Design review of the part built by this model. Coordinates are the model's own, in mm. A direction names the side the tool comes from. Round coordinates to 2 decimals unless told otherwise and drop trailing zeros. Order: outer loops, then holes, each group sorted by start corner. A loop starts at its lowest first (then second) coordinate and runs counter-clockwise, first axis right, second up. Notation, with made-up numbers: (66.25, 34.25) - (110.25, 34.25) arc R27 ccw to (110.25, 55.25) - close; hole circle Ø10 at (28, -9). An arc over 180 degrees is marked (long way). Write item = value, one per line.
from build123d import *

# Parameters (mm, degrees)
F0_W     = 152.4
F0_H     = 152.4
F1_DEPTH = 152.4
F2_R     = 12.7
F4_D     = 38.1
F5_W     = 57.1246
F5_H     = 22.6568
F6_DEPTH = 152.401


with BuildPart() as f1:
    # F0 (on Front) → F1 (new body)
    with BuildSketch(Plane.XZ):
        with Locations((76.2, 76.2)):
            Rectangle(F0_W, F0_H)
    extrude(amount=F1_DEPTH)

    # F2
    f2_edges = [f1.edges().sort_by_distance(p)[0] for p in [
        (76.2, -152.4, 152.4),
        (0, -76.2, 152.4),
        (76.2, 0, 152.4),
        (152.4, -76.2, 152.4),
    ]]
    fillet(f2_edges, radius=F2_R)

    # F4 (through all)
    with Locations(Plane.YZ.offset(152.4)):
        with Locations((-73.099315, 71.219265)):
            Hole(F4_D / 2)

    # F5 (on face) → F6 (cut, through all)
    with BuildSketch(Plane.XZ.offset(152.4)):
        with Locations((66.187836, 65.461391)):
            Rectangle(F5_W, F5_H)
    extrude(amount=-F6_DEPTH, mode=Mode.SUBTRACT)


solid = f1.part
1) We need section A-A on y = -35. Write out the cut boundary in (x, z), and give its area (3 significant figures).
Findings:
outline = (0, 0) - (152.4, 0) - (152.4, 139.7) arc R12.7 ccw to (139.7, 152.4) - (12.7, 152.4) arc R12.7 ccw to (0, 139.7) - close; hole (37.63, 54.13) - (94.75, 54.13) - (94.75, 76.79) - (37.63, 76.79) - close
area = 21,900 mm^2
2) We need section B-B on x = 59. Write out the cut boundary in (y, z), and give its area (3 significant figures).
Findings:
outline = (-152.4, 0) - (0, 0) - (0, 54.13) - (-64.68, 54.13) arc R19.05 cw to (-81.52, 54.13) - (-152.4, 54.13) - close; (-152.4, 76.79) - (-91.32, 76.79) arc R19.05 cw to (-54.88, 76.79) - (0, 76.79) - (0, 139.7) arc R12.7 ccw to (-12.7, 152.4) - (-139.7, 152.4) arc R12.7 ccw to (-152.4, 139.7) - close
area = 19,300 mm^2
3) We need section D-D on y = -74.5. Write out the cut boundary in (x, z), and give its area (3 significant figures).
Findings:
outline = (0, 0) - (152.4, 0) - (152.4, 52.22) - (0, 52.22) - close; (0, 90.22) - (152.4, 90.22) - (152.4, 139.7) arc R12.7 ccw to (139.7, 152.4) - (12.7, 152.4) arc R12.7 ccw to (0, 139.7) - close
area = 17,400 mm^2
4) To check wall thickness, follow L1, parallel to Z at x = 39, y = -123; L2, parallel to Z at x = 37, y = -82; L3, parallel to Y at x = 16, z = 78.5. State the ranges of each line that lie inside material, in increasing order. Write a range as from..to.
Findings:
L1 = 0..54.13, 76.79..152.4
L2 = 0..54.38, 88.06..152.4
L3 = -152.4..-90.7, -55.5..0
5) The part is to be moulded in two halves that separate along Z. For faces 3 (the flat face through (66, -117, 54.133)), 4 (the cylindrical face through (3.62, -77.27, 148.58)), 5 (the flat face through (75, -152.4, 86)), say which applies: released by +Z, released by -Z, zero draft, split by the parting line, or undercut.
Findings:
face_3 = undercut
face_4 = released by +Z
face_5 = zero draft
6) We need section C-C on z = 65. Write out the cut boundary in (x, y), and give its area (3 significant figures).
Findings:
outline = (0, -152.4) - (37.63, -152.4) - (37.63, -91.11) - (0, -91.11) - close; (0, -55.09) - (37.63, -55.09) - (37.63, 0) - (0, 0) - close; (94.75, -152.4) - (152.4, -152.4) - (152.4, -91.11) - (94.75, -91.11) - close; (94.75, -55.09) - (152.4, -55.09) - (152.4, 0) - (94.75, 0) - close
area = 11,100 mm^2
7) For faces 1 (the flat face through (37.626, -117, 65)), 2 (the flat face through (75, -75, 0)), list the 3-axis set-ups (+Z, -Z, +X, -X, +Y, -Y) from which the entire face can be reached by the end or side of a thin tool; tool diameter is ignored.
Findings:
face_1 = +Y, -Y
face_2 = -Z, +X, -X, +Y, -Y
